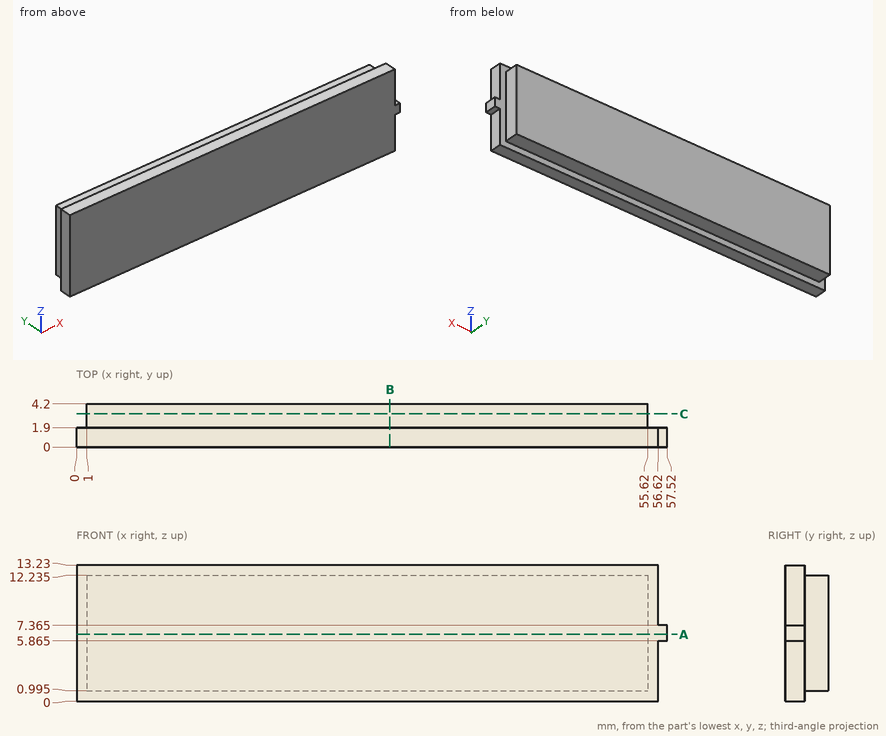
Print and shaded views of the part. All mm, measured from the part's lowest x, y and z. Round coordinates to 2 decimals unless told otherwise and drop trailing zeros. Order: outer loops, then holes, each group sorted by start corner. A loop starts at its lowest first (then second) coordinate and runs counter-clockwise, first axis right, second up.
Q1. Drop flat-ended pins along their axis: pin 1 (1.1 mm diameter, centred on x = 31, y = 3, fed in from +Z) (3 decimals); pin 2 (0.6 mm diameter, centred on y = 0.5, z = 11.5, fed in from +X); pin 3 (1.1 mm diameter, centred on y = 3, z = 8.5, fed in from -X). Give the stop position or say it passes through.
Q2. Slice it at B-B (x = 30.5). Write the cut outline in (y, z) (3 decimals), and give its area (3 significant figures).
Q3. Wall check: L1, parallel to Z at x = 40.5, y = 1.95 (3 decimals); L2, parallel to X at y = 2.65, z = 12; L3, parallel to X at y = 1.85, z = 7.5. Give the ranges that are in metal, low to high.
Q4. Slice it at A-A (z = 6.5). Write the cut outline in (x, y).
Q5. Slice it at C-C (y = 3.25). Write the cut outline in (x, z) (3 decimals), and give its area (3 significant figures).
Results below:
1. pin 1: stops at z = 12.235
1. pin 2: stops at x = 56.62
1. pin 3: stops at x = 1
2. outline: (0, 0) - (1.9, 0) - (1.9, 0.995) - (4.2, 0.995) - (4.2, 12.235) - (1.9, 12.235) - (1.9, 13.23) - (0, 13.23) - close
2. area: 51.0 mm2
3. L1: z = 0.995 to 12.235
3. L2: x = 1 to 55.62
3. L3: x = 0 to 56.62
4. outline: (0, 0) - (57.52, 0) - (57.52, 1.9) - (55.62, 1.9) - (55.62, 4.2) - (1, 4.2) - (1, 1.9) - (0, 1.9) - close
5. outline: (1, 0.995) - (55.62, 0.995) - (55.62, 12.235) - (1, 12.235) - close
5. area: 614 mm2
